Source: three-view drawing plus pictorial views. Frame: mm from the lowest corner of the part. A direction names the side the tool comes from. Round coordinates to 2 decimals unless told otherwise and drop trailing zeros. Order: outer loops, then holes, each group sorted by start corner. A loop starts at its lowest first (then second) coordinate and runs counter-clockwise, first axis right, second up. Notation, with made-up numbers: M 66,40 L 102,40 A13 cw 102,44 Z; hole C 82,66 d8. An arc over 180 degrees is marked long. Return JSON: item names as keys, results as strings. Group by question number.
Q1. Access query for the marked faces 1 and 2. Directions: +Z, -Z, +X, -X, +Y, -Y. A direction counts if a zero-diameter tool reaches every point of the face in a straight line with its end or side. Return the directions, or none.
Q2. Mould query, pull axis Z, two halves, no side actions, for the marked faces 3, 4 and 5. Classes: released by +Z, released by -Z, zero draft, split by the parting line, or undercut.
Q3. Cut plane A-A on y = 21. Output: boundary loops of the cut face in (x, z).
Q4. Contact query for a flat-ended pin moving along its axis: pin 1 (1.5 mm diameter, centred on x = 25.5, z = 47.5, fed in from -Y). Output: stop coordinate, or through.
Q5. Cut plane C-C on z = 39. Output: boundary loops of the cut face in (x, y).
Q6. Cut plane B-B on x = 27. Output: boundary loops of the cut face in (y, z), and give its area (3 significant figures).
Q7. Ray query, probe 1 along Z at (x, y) = (47.5, 49.5); probe 2 along X at (y, z) = (32.5, 18.5); probe 3 along Y at (x, z) = (44, 23.5). Return the intervals inside material, ascending.
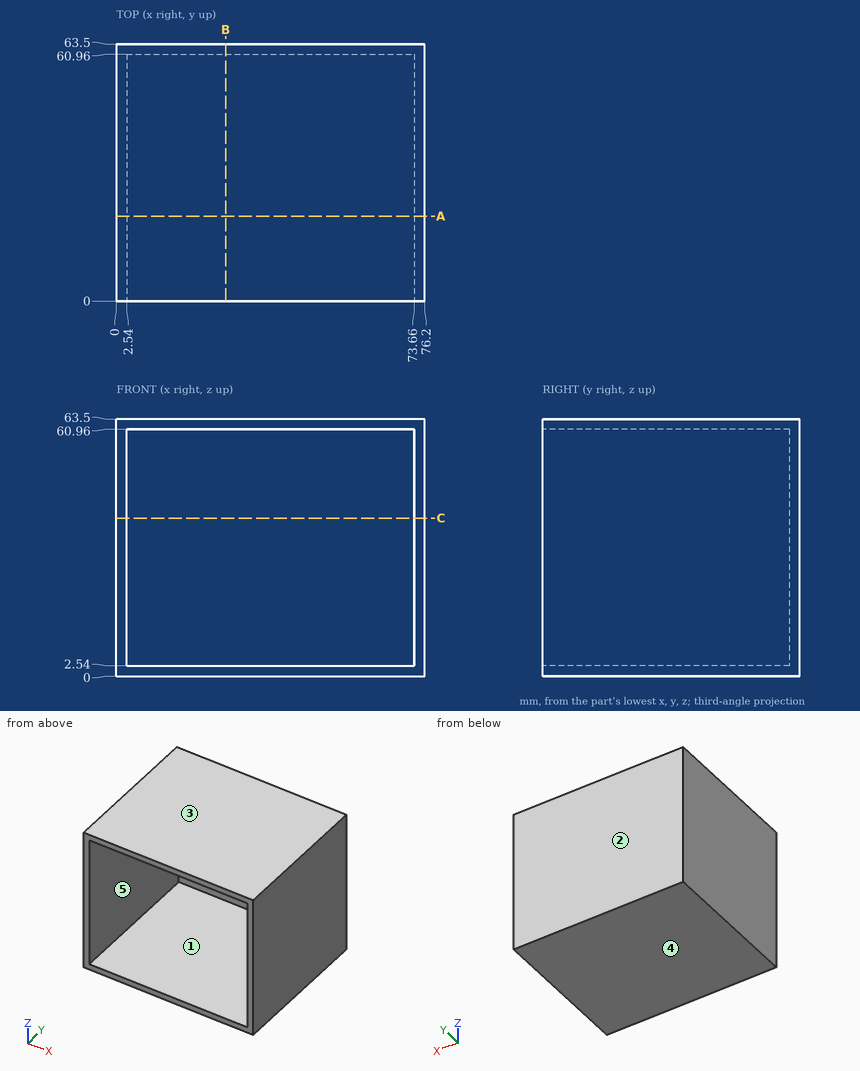
Result sheet:
{
 "1": {"face 1": "-Y", "face 2": "+Z, -Z, +X, -X, +Y"},
 "2": {"face 3": "released by +Z", "face 4": "released by -Z", "face 5": "undercut"},
 "3": {"outline": "M 0,0 L 76.2,0 L 76.2,63.5 L 0,63.5 Z; hole M 2.54,2.54 L 73.66,2.54 L 73.66,60.96 L 2.54,60.96 Z"},
 "4": {"pin 1": "stops at y = 60.96"},
 "5": {"outline": "M 0,0 L 2.54,0 L 2.54,60.96 L 73.66,60.96 L 73.66,0 L 76.2,0 L 76.2,63.5 L 0,63.5 Z"},
 "6": {"outline": "M 0,0 L 63.5,0 L 63.5,63.5 L 0,63.5 L 0,60.96 L 60.96,60.96 L 60.96,2.54 L 0,2.54 Z", "area": "471 mm²"},
 "7": {"probe 1": "z = 0 to 2.54, 60.96 to 63.5", "probe 2": "x = 0 to 2.54, 73.66 to 76.2", "probe 3": "y = 60.96 to 63.5"}
}
